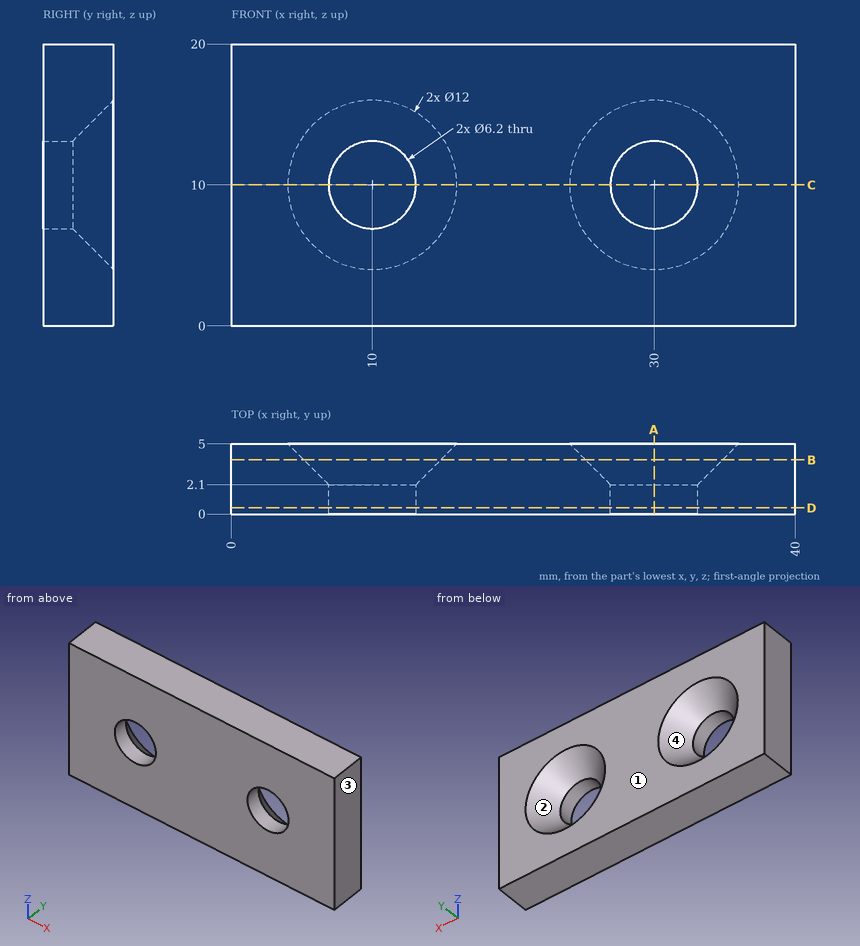
Input: dimensioned drawing with shaded views. Units: mm. Origin: part minimum x, y, z. Round coordinates to 2 decimals unless told otherwise and drop trailing zeros. Order: outer loops, then holes, each group sorted by start corner. A loop starts at its lowest first (then second) coordinate and runs counter-clockwise, first axis right, second up. Notation, with made-up numbers: (29.5, 38) - (39.5, 38) arc R30 cw to (39.5, 69) - close; hole circle Ø10 at (71, 40). An arc over 180 degrees is marked (long way). Use CSV: the item, a comma, the result in double quotes. Start each with the question number.
Q1. Section query B-B (y = 3.85). Return loops of the section in (x, z), and give its area (3 significant figures).
Q2. Section query A-A (x = 30). Return loops of the section in (y, z), and give its area (3 significant figures).
Q3. First-contact query: pin 1 (5.5 mm diameter, centred on x = 30, z = 10, fed in from -Y). Flat tip, straight axial feed; report the tip coordinate or a pass-through.
Q4. Mould query, pull axis X, two halves, no side actions, for the marked faces 1, 2, 3 and 4. Classes: +X half, -X half, draft (parallel to the pull), parting line (faces both ways), or undercut.
Q5. Section query C-C (z = 10). Return loops of the section in (x, y), and give its area (3 significant figures).
Q6. Section query D-D (y = 0.45). Return loops of the section in (x, z), and give its area (3 significant figures).
Q7. Material intervals for line 1 along X through (y, z) = (0.4, 10); line 2 along Z through (x, y) = (30, 1.05); line 3 along X through (y, z) = (4.35, 8.75), sorted ascending. Write a range as from..to.
Result set:
1,outline,"(0, 0) - (40, 0) - (40, 20) - (0, 20) - close; hole circle Ø9.7 at (10, 10); hole circle Ø9.7 at (30, 10)"
1,area,"652 mm2"
2,outline,"(0, 0) - (5, 0) - (5, 4) - (2.1, 6.9) - (0, 6.9) - close; (0, 13.1) - (2.1, 13.1) - (5, 16) - (5, 20) - (0, 20) - close"
2,area,"60.6 mm2"
3,pin 1,"passes through"
4,face 1,"draft"
4,face 2,"undercut"
4,face 3,"+X half"
4,face 4,"undercut"
5,outline,"(0, 0) - (6.9, 0) - (6.9, 2.1) - (4, 5) - (0, 5) - close; (13.1, 0) - (26.9, 0) - (26.9, 2.1) - (24, 5) - (16, 5) - (13.1, 2.1) - close; (33.1, 0) - (40, 0) - (40, 5) - (36, 5) - (33.1, 2.1) - close"
5,area,"121 mm2"
6,outline,"(0, 0) - (40, 0) - (40, 20) - (0, 20) - close; hole circle Ø6.2 at (10, 10); hole circle Ø6.2 at (30, 10)"
6,area,"740 mm2"
7,line 1,"x = 0..6.9, 13.1..26.9, 33.1..40"
7,line 2,"z = 0..6.9, 13.1..20"
7,line 3,"x = 0..4.8, 15.2..24.8, 35.2..40"
